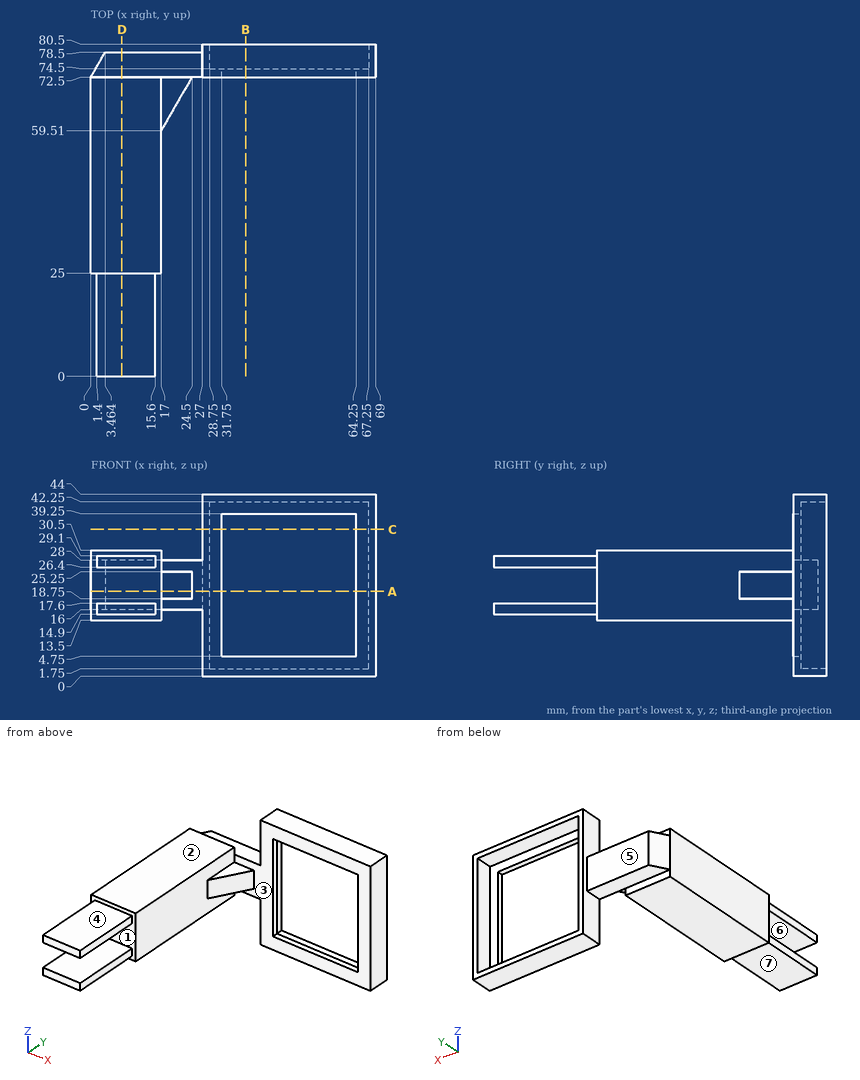
Print and shaded views of the part. All mm, measured from the part's lowest x, y and z. A direction names the side the tool comes from. Coordinates: 2 decimals unless noted, no trailing zeros. Order: outer loops, then holes, each group sorted by start corner. A loop starts at its lowest first (then second) coordinate and runs counter-clockwise, first axis right, second up. Notation, with made-up numbers: (11, -31) - (21, -31) arc R25 ccw to (21, -17) - close; hole circle Ø1 at (15, 61.5). An arc over 180 degrees is marked (long way). Return JSON: item names as keys, results as strings. Group by question number.
Item 1: Cut at C-C (z = 35.5). List the corners of the cut face in (x, y), plus the area to 3 significant figures.
Item 2: Which spindle directions (+Z, -Z, +X, -X, +Y, -Y) get a long thin tool onto all of the face, cutting with end or side? Do the marked faces 4, 5, 6 and 7. Say none if no direction does.
Item 3: Cut at D-D (x = 7.5). List the corners of the cut face in (y, z).
Item 4: Pin check, flat tips, straight feed: pin 1 (0.8 mm diameter, centred on y = 12, z = 16.5, fed in from +X); pin 2 (7 mm diameter, centred on x = 6.5, y = 13, fed in from -Z); pin 3 (15.5 mm diameter, centred on x = 8, y = 8, fed in from +Z); pin 4 (5 mm diameter, centred on x = 40, y = 77, fed in from -Z). Stop position of each tip, or through.
Item 5: Pull direction Z, two halves, no side cores. Call the marked faces 1, 2 and 3: pulls with the +Z half, pulls with the -Z half, needs draft (parallel to the pull), parting line crosses it, or undercut.
Item 6: Cut at B-B (x = 37.5). List the corners of the cut face in (y, z), plus the area to 3 significant figures.
Item 7: Drill centre lines: probe 1 along Y at (x, z) = (66, 23.5); probe 2 along Y at (x, z) = (28, 39.5); probe 3 along Z at (x, y) = (10, 67). Where is each one in solid material? Low to high. Write a range as from..to.
Item 8: Cut at A-A (z = 20.5). List the corners of the cut face in (x, y).
Check values:
{
 "1": {"outline": "(27, 72.5) - (31.75, 72.5) - (31.75, 74.5) - (28.75, 74.5) - (28.75, 80.5) - (27, 80.5) - close; (64.25, 72.5) - (69, 72.5) - (69, 80.5) - (67.25, 80.5) - (67.25, 74.5) - (64.25, 74.5) - close", "area": "40.0 mm2"},
 "2": {"face 4": "+Z, +X, -X, -Y", "face 5": "+Z, -Z, -X, +Y", "face 6": "+X, -X, -Y", "face 7": "-Z, +X, -X, -Y"},
 "3": {"outline": "(0, 14.9) - (25, 14.9) - (25, 13.5) - (72.5, 13.5) - (72.5, 16) - (78.5, 16) - (78.5, 28) - (72.5, 28) - (72.5, 30.5) - (25, 30.5) - (25, 29.1) - (0, 29.1) - (0, 26.4) - (25, 26.4) - (25, 17.6) - (0, 17.6) - close"},
 "4": {"pin 1": "stops at x = 15.6", "pin 2": "stops at z = 14.9", "pin 3": "stops at z = 29.1", "pin 4": "stops at z = 0"},
 "5": {"face 1": "undercut", "face 2": "pulls with the +Z half", "face 3": "needs draft"},
 "6": {"outline": "(72.5, 0) - (80.5, 0) - (80.5, 1.75) - (74.5, 1.75) - (74.5, 4.75) - (72.5, 4.75) - close; (72.5, 39.25) - (74.5, 39.25) - (74.5, 42.25) - (80.5, 42.25) - (80.5, 44) - (72.5, 44) - close", "area": "40.0 mm2"},
 "7": {"probe 1": "y = 72.5..74.5", "probe 2": "y = 72.5..80.5", "probe 3": "z = 13.5..30.5"},
 "8": {"outline": "(0, 25) - (17, 25) - (17, 59.51) - (24.5, 72.5) - (31.75, 72.5) - (31.75, 74.5) - (28.75, 74.5) - (28.75, 80.5) - (27, 80.5) - (27, 78.5) - (3.46, 78.5) - (0, 72.5) - close; (64.25, 72.5) - (69, 72.5) - (69, 80.5) - (67.25, 80.5) - (67.25, 74.5) - (64.25, 74.5) - close"}
}
